For this review, take the finished solid that the model builds, in its own axes (mm). A direction names the side the tool comes from. Coordinates: 2 decimals unless noted, no trailing zeros. Write each loop counter-clockwise with the first axis right and the second up, starting at its lowest first coordinate (ties: lowest second). Pieces come first, ordered by that corner, then holes. Notation, with made-up numbers: M -9.75,-4.75 L 48.25,-4.75 A21 ccw 48.25,12.25 Z; hole C -6.5,-1.5 d4. An arc over 180 degrees is marked long. Return JSON: item names as keys, results as strings.
```python
from build123d import *

# Parameters (mm, degrees)
SKETCH1_R           = 1.5
BOSS_EXTRUDE1_DEPTH = 5


with BuildPart() as part:
    # Sketch1 → Boss-Extrude1 (new body)
    with BuildSketch(Plane.XY):
        with BuildLine():
            Line((5, -5), (5, -111))
            ThreePointArc((5, -111), (0, -116), (-5, -111))
            Line((-5, -111), (-5, -5))
            Line((-5, -5), (-111, -5))
            ThreePointArc((-111, -5), (-116, 0), (-111, 5))
            Line((-111, 5), (-5, 5))
            Line((-5, 5), (-5, 111))
            ThreePointArc((-5, 111), (0, 116), (5, 111))
            Line((5, 111), (5, 5))
            Line((5, 5), (111, 5))
            ThreePointArc((111, 5), (116, 0), (111, -5))
            Line((111, -5), (5, -5))
        make_face()
        Circle(SKETCH1_R, mode=Mode.SUBTRACT)
        with Locations((0, -111)):
            Circle(SKETCH1_R, mode=Mode.SUBTRACT)
        with Locations((-111, 0)):
            Circle(SKETCH1_R, mode=Mode.SUBTRACT)
        with Locations((0, 111)):
            Circle(SKETCH1_R, mode=Mode.SUBTRACT)
        with Locations((111, 0)):
            Circle(SKETCH1_R, mode=Mode.SUBTRACT)
    extrude(amount=BOSS_EXTRUDE1_DEPTH)


solid = part.part
```
1. Wall thickness on L1, parallel to Y at x = 0, z = 1.85; L2, parallel to X at y = 111, z = 2.9; L3, parallel to X at y = 104, z = 2.95: over which ranges is each line inside the solid? List them lowest first. Write a range as from..to.
Checks:
{"L1": "-116..-112.5, -109.5..-1.5, 1.5..109.5, 112.5..116", "L2": "-5..-1.5, 1.5..5", "L3": "-5..5"}
2. Clearance check with flat-ended pins moving along their axes: pin 1 Ø1.5 at (y, z) = (58.5, 3.5) entering from -X; pin 2 Ø5 at (x, y) = (8.5, -64.5) entering from -Z; pin 3 Ø1.5 at (x, z) = (64, 2) entering from -Y; pin 4 Ø1.5 at (x, z) = (-31.5, 2) entering from +Y. State where each tip first meets the part, or that it passes through.
Checks:
{"pin 1": "x = -5", "pin 2": "through", "pin 3": "y = -5", "pin 4": "y = 5"}
3. We need section B-B (x = -80.5). State the section outline as (y, z) points, plus the area to 3 significant figures.
Checks:
{"outline": "M -5,0 L 5,0 L 5,5 L -5,5 Z", "area": "50.0 mm2"}
4. For faces 1 (the face through (-5, -59, 2)), 2 (the face through (-59, 5, 2)), 3 (the face through (5, 59, 2)), list the 3-axis set-ups (+Z, -Z, +X, -X, +Y, -Y) from which the entire face can be reached by the end or side of a thin tool; tool diameter is ignored.
Checks:
{"face 1": "+Z, -Z, -X, -Y", "face 2": "+Z, -Z, -X, +Y", "face 3": "+Z, -Z, +X, +Y"}
5. We need section A-A (z = 1.15). State the section outline as (x, y) points.
Checks:
{"outline": "M -111,-5 L -5,-5 L -5,-111 A5 ccw 5,-111 L 5,-5 L 111,-5 A5 ccw 111,5 L 5,5 L 5,111 A5 ccw -5,111 L -5,5 L -111,5 A5 ccw Z; hole C -111,0 d3; hole C 0,-111 d3; hole C 0,0 d3; hole C 0,111 d3; hole C 111,0 d3"}
